Job drawing, mm, ordinate dimensions from the low corner. One solid piece. Give positions to 0.01 mm unless a question says otherwise; leave off trailing zeros. Loops run counter-clockwise (first coordinate to the right, second up) from the corner with the lowest first, then second, coordinate; pieces in that order, holes last.
Item 1: Probe probe 1 along X at (y, z) = (0.7, 428) (1 decimal); probe 2 along X at (y, z) = (2.05, 32) (1 decimal); probe 3 along Z at (x, y) = (472, 0.7) (1 decimal). List the from-to ranges inside material, lowest first.
Item 2: Saw through at D-D on z = 548.5. Give the cut face in (x, y), plus the area to 3 significant figures.
Item 3: Saw through at B-B on y = 4. Give the number of separate pieces and of enclosed holes in the cut face, plus the area to 3 significant figures.
Item 4: Saw through at A-A on z = 335. Give the cut face in (x, y).
Item 5: Drop flat-ended pins along their axis: P1, Ø8, axis at x = 478.5, z = 231, coming from the -Y side; P2, Ø1.5, axis at x = 133, y = 2.5, coming from the -Z side; P3, Ø1, axis at y = 1, z = 75.5, coming from the -X side; P4, Ø1.5, axis at x = 131, y = 2.5, coming from the -Z side. Give the stop position or say it passes through.
Item 6: Saw through at C-C on x = 478.5. Give the cut face in (y, z).
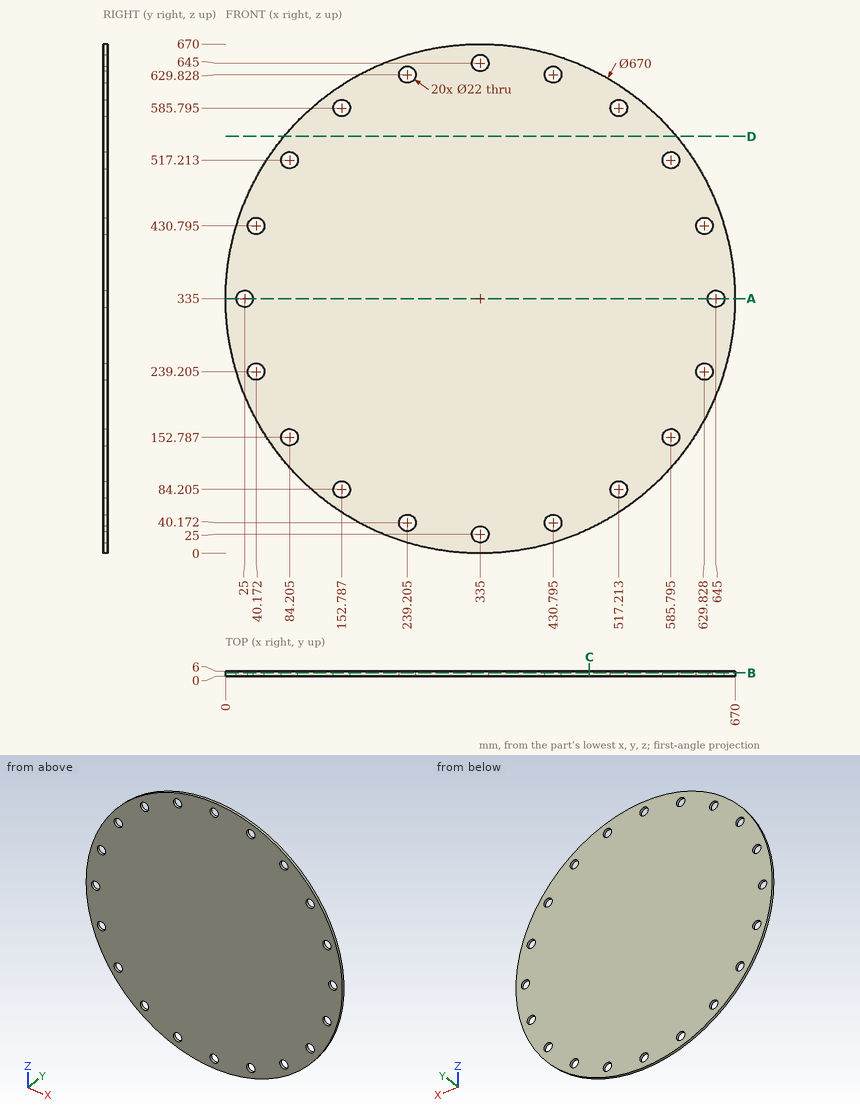
Results below:
1. probe 1: x = 13.2 to 29.5, 50.8 to 619.2, 640.5 to 656.8
1. probe 2: x = 192.1 to 231.8, 246.6 to 326.5, 343.5 to 423.4, 438.2 to 477.9
1. probe 3: z = 29.3 to 640.7
2. outline: (76.85, 0) - (593.15, 0) - (593.15, 6) - (76.85, 6) - close
2. area: 3,100 mm2
3. separate pieces: 1
3. enclosed holes: 20
3. area: 345,000 mm2
4. outline: (0, 0) - (14, 0) - (14, 6) - (0, 6) - close; (36, 0) - (634, 0) - (634, 6) - (36, 6) - close; (656, 0) - (670, 0) - (670, 6) - (656, 6) - close
5. P1: stops at y = 0
5. P2: stops at z = 67.19
5. P3: stops at x = 122.53
5. P4: stops at z = 68.7
6. outline: (0, 32.29) - (6, 32.29) - (6, 637.71) - (0, 637.71) - close
